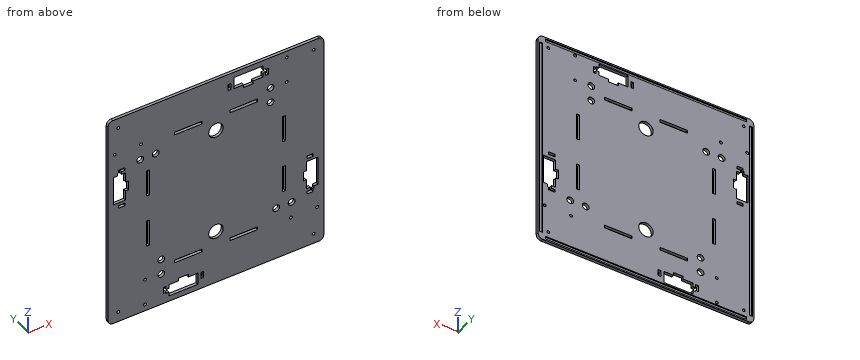
from build123d import *

# Parameters (mm, degrees)
SKETCH1_W           = 224.4
SKETCH1_H           = 224.4
SKETCH1_R           = 1.5
SKETCH1_W_2         = 28.88
SKETCH1_H_2         = 3
SKETCH1_W_3         = 3
SKETCH1_H_3         = 27.68
BOSS_EXTRUDE1_DEPTH = 3
FILLET1_R           = 5
SKETCH2_W           = 209.4
SKETCH2_H           = 3
SKETCH2_W_2         = 3
SKETCH2_H_2         = 209.4
CUT_EXTRUDE1_DEPTH  = 1
CUT_EXTRUDE3_DEPTH  = 4
CUT_EXTRUDE4_REACH  = 5
SKETCH4_R           = 1.5
SKETCH5_W           = 3
SKETCH5_H           = 6.55
SKETCH5_W_2         = 6.55
SKETCH5_H_2         = 3
CUT_EXTRUDE5_DEPTH  = 4
SKETCH6_R           = 3.5
CUT_EXTRUDE6_DEPTH  = 4
SKETCH13_R          = 7.5
CUT_EXTRUDE10_DEPTH = 4


with BuildPart() as part:
    # Sketch1 → Boss-Extrude1 (new body)
    with BuildSketch(Plane(origin=(0, 0, 0), x_dir=(1, 0, 0), z_dir=(0, 1, 0))):
        with Locations((112.2, 112.2)):
            Rectangle(SKETCH1_W, SKETCH1_H)
        with Locations((213.9, 10.5)):
            Circle(SKETCH1_R, mode=Mode.SUBTRACT)
        with Locations((213.9, 213.9)):
            Circle(SKETCH1_R, mode=Mode.SUBTRACT)
        with Locations((10.5, 10.5)):
            Circle(SKETCH1_R, mode=Mode.SUBTRACT)
        with Locations((10.5, 213.9)):
            Circle(SKETCH1_R, mode=Mode.SUBTRACT)
        with Locations((83.32, 41.5)):
            Rectangle(SKETCH1_W_2, SKETCH1_H_2, mode=Mode.SUBTRACT)
        with Locations((141.08, 41.5)):
            Rectangle(SKETCH1_W_2, SKETCH1_H_2, mode=Mode.SUBTRACT)
        with Locations((141.08, 182.9)):
            Rectangle(SKETCH1_W_2, SKETCH1_H_2, mode=Mode.SUBTRACT)
        with Locations((83.32, 182.9)):
            Rectangle(SKETCH1_W_2, SKETCH1_H_2, mode=Mode.SUBTRACT)
        with Locations((41.5, 84.52)):
            Rectangle(SKETCH1_W_3, SKETCH1_H_3, mode=Mode.SUBTRACT)
        with Locations((41.5, 139.88)):
            Rectangle(SKETCH1_W_3, SKETCH1_H_3, mode=Mode.SUBTRACT)
        with Locations((182.9, 139.88)):
            Rectangle(SKETCH1_W_3, SKETCH1_H_3, mode=Mode.SUBTRACT)
        with Locations((182.9, 84.52)):
            Rectangle(SKETCH1_W_3, SKETCH1_H_3, mode=Mode.SUBTRACT)
    extrude(amount=BOSS_EXTRUDE1_DEPTH)

    # Fillet1
    fillet1_edges = [part.edges().sort_by_distance(p)[0] for p in [
        (0, 1.5, -224.4),
        (224.4, 1.5, -224.4),
        (224.4, 1.5, 0),
        (0, 1.5, 0),
    ]]
    fillet(fillet1_edges, radius=FILLET1_R)

    # Sketch2 → Cut-Extrude1 (cut)
    with BuildSketch(Plane(origin=(0, 3, 0), x_dir=(1, 0, 0), z_dir=(0, 1, 0))):
        with Locations((112.2, 3)):
            Rectangle(SKETCH2_W, SKETCH2_H)
        with Locations((221.4, 112.2)):
            Rectangle(SKETCH2_W_2, SKETCH2_H_2)
        with Locations((112.2, 221.4)):
            Rectangle(SKETCH2_W, SKETCH2_H)
        with Locations((3, 112.2)):
            Rectangle(SKETCH2_W_2, SKETCH2_H_2)
    extrude(amount=-CUT_EXTRUDE1_DEPTH, mode=Mode.SUBTRACT)

    # Sketch3 → Cut-Extrude3 (cut, through all)
    with BuildSketch(Plane(origin=(0, 3, 0), x_dir=(1, 0, 0), z_dir=(0, 1, 0))):
        Polygon((131, 18.15), (131, 5.85), (161, 5.85), (161, 9.95), (164, 9.95), (164, 14.05), (161, 14.05), (161, 18.15), (151, 18.15), (151, 21.15), (141, 21.15), (141, 18.15), align=None)
        Polygon((18.15, 93.4), (5.85, 93.4), (5.85, 63.4), (9.95, 63.4), (9.95, 60.4), (14.05, 60.4), (14.05, 63.4), (18.15, 63.4), (18.15, 73.4), (21.15, 73.4), (21.15, 83.4), (18.15, 83.4), align=None)
        Polygon((93.4, 206.25), (93.4, 218.55), (63.4, 218.55), (63.4, 214.45), (60.4, 214.45), (60.4, 210.35), (63.4, 210.35), (63.4, 206.25), (73.4, 206.25), (73.4, 203.25), (83.4, 203.25), (83.4, 206.25), align=None)
        Polygon((206.25, 131), (218.55, 131), (218.55, 161), (214.45, 161), (214.45, 164), (210.35, 164), (210.35, 161), (206.25, 161), (206.25, 151), (203.25, 151), (203.25, 141), (206.25, 141), align=None)
    extrude(amount=-CUT_EXTRUDE3_DEPTH, mode=Mode.SUBTRACT)

    # Sketch4 → Cut-Extrude4 (cut, up to next)
    with BuildSketch(Plane(origin=(0, 3, 0), x_dir=(1, 0, 0), z_dir=(0, 1, 0)), mode=Mode.PRIVATE) as cut_extrude4_sk1:
        with Locations((38.54888627, 217.45)):
            Circle(SKETCH4_R)
    cut_extrude4_tool1 = extrude(cut_extrude4_sk1.sketch, amount=-CUT_EXTRUDE4_REACH, mode=Mode.PRIVATE) & part.part
    add(cut_extrude4_tool1.solids().sort_by_distance((38.548886, 3, -217.45))[0], mode=Mode.SUBTRACT)
    # Sketch4 → Cut-Extrude4 (cut, up to next)
    with BuildSketch(Plane(origin=(0, 3, 0), x_dir=(1, 0, 0), z_dir=(0, 1, 0)), mode=Mode.PRIVATE) as cut_extrude4_sk2:
        with Locations((38.54888627, 190.15)):
            Circle(SKETCH4_R)
    cut_extrude4_tool2 = extrude(cut_extrude4_sk2.sketch, amount=-CUT_EXTRUDE4_REACH, mode=Mode.PRIVATE) & part.part
    add(cut_extrude4_tool2.solids().sort_by_distance((38.548886, 3, -190.15))[0], mode=Mode.SUBTRACT)
    # Sketch4 → Cut-Extrude4 (cut, up to next)
    with BuildSketch(Plane(origin=(0, 3, 0), x_dir=(1, 0, 0), z_dir=(0, 1, 0)), mode=Mode.PRIVATE) as cut_extrude4_sk3:
        with Locations((217.45, 185.85111373)):
            Circle(SKETCH4_R)
    cut_extrude4_tool3 = extrude(cut_extrude4_sk3.sketch, amount=-CUT_EXTRUDE4_REACH, mode=Mode.PRIVATE) & part.part
    add(cut_extrude4_tool3.solids().sort_by_distance((217.45, 3, -185.851114))[0], mode=Mode.SUBTRACT)
    # Sketch4 → Cut-Extrude4 (cut, up to next)
    with BuildSketch(Plane(origin=(0, 3, 0), x_dir=(1, 0, 0), z_dir=(0, 1, 0)), mode=Mode.PRIVATE) as cut_extrude4_sk4:
        with Locations((190.15, 185.85111373)):
            Circle(SKETCH4_R)
    cut_extrude4_tool4 = extrude(cut_extrude4_sk4.sketch, amount=-CUT_EXTRUDE4_REACH, mode=Mode.PRIVATE) & part.part
    add(cut_extrude4_tool4.solids().sort_by_distance((190.15, 3, -185.851114))[0], mode=Mode.SUBTRACT)
    # Sketch4 → Cut-Extrude4 (cut, up to next)
    with BuildSketch(Plane(origin=(0, 3, 0), x_dir=(1, 0, 0), z_dir=(0, 1, 0)), mode=Mode.PRIVATE) as cut_extrude4_sk5:
        with Locations((185.85111373, 6.95)):
            Circle(SKETCH4_R)
    cut_extrude4_tool5 = extrude(cut_extrude4_sk5.sketch, amount=-CUT_EXTRUDE4_REACH, mode=Mode.PRIVATE) & part.part
    add(cut_extrude4_tool5.solids().sort_by_distance((185.851114, 3, -6.95))[0], mode=Mode.SUBTRACT)
    # Sketch4 → Cut-Extrude4 (cut, up to next)
    with BuildSketch(Plane(origin=(0, 3, 0), x_dir=(1, 0, 0), z_dir=(0, 1, 0)), mode=Mode.PRIVATE) as cut_extrude4_sk6:
        with Locations((185.85111373, 34.25)):
            Circle(SKETCH4_R)
    cut_extrude4_tool6 = extrude(cut_extrude4_sk6.sketch, amount=-CUT_EXTRUDE4_REACH, mode=Mode.PRIVATE) & part.part
    add(cut_extrude4_tool6.solids().sort_by_distance((185.851114, 3, -34.25))[0], mode=Mode.SUBTRACT)
    # Sketch4 → Cut-Extrude4 (cut, up to next)
    with BuildSketch(Plane(origin=(0, 3, 0), x_dir=(1, 0, 0), z_dir=(0, 1, 0)), mode=Mode.PRIVATE) as cut_extrude4_sk7:
        with Locations((6.95, 38.54888627)):
            Circle(SKETCH4_R)
    cut_extrude4_tool7 = extrude(cut_extrude4_sk7.sketch, amount=-CUT_EXTRUDE4_REACH, mode=Mode.PRIVATE) & part.part
    add(cut_extrude4_tool7.solids().sort_by_distance((6.95, 3, -38.548886))[0], mode=Mode.SUBTRACT)
    # Sketch4 → Cut-Extrude4 (cut, up to next)
    with BuildSketch(Plane(origin=(0, 3, 0), x_dir=(1, 0, 0), z_dir=(0, 1, 0)), mode=Mode.PRIVATE) as cut_extrude4_sk8:
        with Locations((34.25, 38.54888627)):
            Circle(SKETCH4_R)
    cut_extrude4_tool8 = extrude(cut_extrude4_sk8.sketch, amount=-CUT_EXTRUDE4_REACH, mode=Mode.PRIVATE) & part.part
    add(cut_extrude4_tool8.solids().sort_by_distance((34.25, 3, -38.548886))[0], mode=Mode.SUBTRACT)

    # Sketch5 → Cut-Extrude5 (cut, through all)
    with BuildSketch(Plane(origin=(0, 3, 0), x_dir=(1, 0, 0), z_dir=(0, 1, 0))):
        with Locations((126.5, 14.325)):
            Rectangle(SKETCH5_W, SKETCH5_H)
        with Locations((165.5, 14.325)):
            Rectangle(SKETCH5_W, SKETCH5_H)
        with Locations((14.325, 97.9)):
            Rectangle(SKETCH5_W_2, SKETCH5_H_2)
        with Locations((14.325, 58.9)):
            Rectangle(SKETCH5_W_2, SKETCH5_H_2)
        with Locations((97.9, 210.075)):
            Rectangle(SKETCH5_W, SKETCH5_H)
        with Locations((58.9, 210.075)):
            Rectangle(SKETCH5_W, SKETCH5_H)
        with Locations((210.075, 126.5)):
            Rectangle(SKETCH5_W_2, SKETCH5_H_2)
        with Locations((210.075, 165.5)):
            Rectangle(SKETCH5_W_2, SKETCH5_H_2)
    extrude(amount=-CUT_EXTRUDE5_DEPTH, mode=Mode.SUBTRACT)

    # Sketch6 → Cut-Extrude6 (cut, through all)
    with BuildSketch(Plane(origin=(0, 3, 0), x_dir=(1, 0, 0), z_dir=(0, 1, 0))):
        with Locations((169.05, 33.5)):
            Circle(SKETCH6_R)
        with Locations((169.05, 49.5)):
            Circle(SKETCH6_R)
        with Locations((33.5, 55.35)):
            Circle(SKETCH6_R)
        with Locations((49.5, 55.35)):
            Circle(SKETCH6_R)
        with Locations((55.35, 190.9)):
            Circle(SKETCH6_R)
        with Locations((55.35, 174.9)):
            Circle(SKETCH6_R)
        with Locations((190.9, 169.05)):
            Circle(SKETCH6_R)
        with Locations((174.9, 169.05)):
            Circle(SKETCH6_R)
    extrude(amount=-CUT_EXTRUDE6_DEPTH, mode=Mode.SUBTRACT)

    # Sketch13 → Cut-Extrude10 (cut, through all)
    with BuildSketch(Plane(origin=(0, 3, 0), x_dir=(1, 0, 0), z_dir=(0, 1, 0))):
        with Locations((112.2, 56.350000001)):
            Circle(SKETCH13_R)
        with Locations((112.2, 168.049999999)):
            Circle(SKETCH13_R)
    extrude(amount=-CUT_EXTRUDE10_DEPTH, mode=Mode.SUBTRACT)


solid = part.part
Input: part model. Units: mm. Frame: model coordinates. Give positions to 0.01 mm unless a question says otherwise; leave off trailing zeros. Order: outer loops, then holes, each group sorted by start corner. A loop starts at its lowest first (then second) coordinate and runs counter-clockwise, first axis right, second up. Notation, with made-up numbers: (-32.75, 69.5) -> (-8.75, 69.5) arc R29 cw to (-8.75, 102.5) -> close; hole circle Ø1 at (-11, -33). An arc over 180 degrees is marked (long way). Use one line per item in the form item = value.
1) Line query: probe 1 along X at (y, z) = (1, -56); probe 2 along Z at (x, y) = (82, 1.6); probe 3 along Z at (x, y) = (45, 2.15). Output: solid intervals per line, ascending.
Response values:
probe_1 = 0 to 30.06, 36.94 to 46.06, 52.94 to 104.71, 119.69 to 224.4
probe_2 = -224.4 to -218.55, -203.25 to -184.4, -181.4 to -43, -40 to 0
probe_3 = -224.4 to -222.9, -219.9 to -4.5, -1.5 to 0
2) Section B-B, the plane x = 87.5. Return loops of the section in (y, z), and give its area (3 significant figures).
Response values:
outline = (0, -224.4) -> (3, -224.4) -> (3, -222.9) -> (2, -222.9) -> (2, -219.9) -> (3, -219.9) -> (3, -218.55) -> (0, -218.55) -> close; (0, -206.25) -> (3, -206.25) -> (3, -184.4) -> (0, -184.4) -> close; (0, -181.4) -> (3, -181.4) -> (3, -43) -> (0, -43) -> close; (0, -40) -> (3, -40) -> (3, -4.5) -> (2, -4.5) -> (2, -1.5) -> (3, -1.5) -> (3, 0) -> (0, 0) -> close
area = 612 mm^2
3) Section A-A, the plane z = -90. Return loops of the section in (x, y).
Response values:
outline = (0, 0) -> (5.85, 0) -> (5.85, 3) -> (4.5, 3) -> (4.5, 2) -> (1.5, 2) -> (1.5, 3) -> (0, 3) -> close; (18.15, 0) -> (40, 0) -> (40, 3) -> (18.15, 3) -> close; (43, 0) -> (181.4, 0) -> (181.4, 3) -> (43, 3) -> close; (184.4, 0) -> (224.4, 0) -> (224.4, 3) -> (222.9, 3) -> (222.9, 2) -> (219.9, 2) -> (219.9, 3) -> (184.4, 3) -> close
4) Section C-C, the plane y = 0.45. Count the separate pieces of the cut face and the enclosed holes in it, and give its area (3 significant figures).
Response values:
separate_pieces = 1
enclosed_holes = 38
area = 47,100 mm^2
